Verification items for the finished model (mm, model axes). A direction names the side the tool comes from. Round coordinates to 2 decimals unless told otherwise and drop trailing zeros. Loops run counter-clockwise (first coordinate to the right, second up) from the corner with the lowest first, then second, coordinate; pieces in that order, holes last. Notation, with made-up numbers: (20, 54) -> (62, 54) arc R31 cw to (62, 79) -> close; hole circle Ø11 at (-35, -30). An arc over 180 degrees is marked (long way). Write item = value, one per line.
```python
from build123d import *

# Parameters (mm, degrees)
F4_DEPTH = 8
F2_R     = 3.171744
F5_DEPTH = 25
F0_R     = 3.171744
F6_DEPTH = 25


with BuildPart() as f4:
    # F3 (on Front) → F4 (new body)
    with BuildSketch(Plane.XZ):
        with BuildLine():
            Line((-59.009388, 95.835626), (0, -18.867213))
            Line((0, -18.867213), (59.009388, 95.835626))
            ThreePointArc((59.009388, 95.835626), (55.394876, 108.451405), (42.578131, 105.631188))
            Line((42.578131, 105.631188), (0, 23.474881))
            Line((0, 23.474881), (-42.578131, 105.631188))
            ThreePointArc((-42.578131, 105.631188), (-55.394876, 108.451405), (-59.009388, 95.835626))
        make_face()
    extrude(amount=F4_DEPTH)

    # F2 (on Front) → F5 (cut)
    with BuildSketch(Plane.XZ):
        with Locations((-50.368942, 99.972241)):
            Circle(F2_R)
        with Locations((50.368942, 99.972241)):
            Circle(F2_R)
    extrude(amount=F5_DEPTH, mode=Mode.SUBTRACT)

    # F0 (on Front) → F6 (cut)
    with BuildSketch(Plane.XZ):
        Circle(F0_R)
    extrude(amount=F6_DEPTH, mode=Mode.SUBTRACT)


solid = f4.part
```
(1) Sectioned sample at A-A, the plane z = 92. Record the cut outline in (x, y), and give its area (3 significant figures).
Filled sheet:
outline = (-57.04, -8) -> (-35.51, -8) -> (-35.51, 0) -> (-57.04, 0) -> close; (35.51, -8) -> (57.04, -8) -> (57.04, 0) -> (35.51, 0) -> close
area = 344 mm2
(2) Sectioned sample at D-D, the plane x = 6. Record the cut outline in (y, z), and give its area (3 significant figures).
Filled sheet:
outline = (-8, -7.2) -> (0, -7.2) -> (0, 35.05) -> (-8, 35.05) -> close
area = 338 mm2
(3) Sectioned sample at B-B, the plane y = -1.25. Record the cut outline in (x, z).
Filled sheet:
outline = (-59.01, 95.84) -> (0, -18.87) -> (59.01, 95.84) arc R9.58 ccw to (42.58, 105.63) -> (0, 23.47) -> (-42.58, 105.63) arc R9.58 ccw to start; hole circle Ø6.34 at (-50.37, 99.97); hole circle Ø6.34 at (0, 0); hole circle Ø6.34 at (50.37, 99.97)
(4) Go/stop test with flat-tipped pins: pin 1 Ø7.5 at (x, z) = (50.37, 99.97) entering from +Y; pin 2 Ø1.5 at (y, z) = (-6, 24) entering from +X; pin 3 Ø5 at (x, z) = (-50.37, 99.97) entering from -Y; pin 4 Ø3 at (y, z) = (-3.5, 37) entering from +X. Record where each tip stops, or that it passes through.
Filled sheet:
pin_1 = 0
pin_2 = 22.44
pin_3 = through
pin_4 = 29.51
(5) Material ranges on probe 1 along X at (y, z) = (-0.5, 35); probe 2 along X at (y, z) = (-0.75, 44); probe 3 along Z at (x, y) = (-5, -3), recorded low to high. Write a range as from..to.
Filled sheet:
probe_1 = -27.71..-5.97, 5.97..27.71
probe_2 = -32.34..-10.64, 10.64..32.34
probe_3 = -9.15..33.12
(6) Sectioned sample at C-C, the plane z = 75. Record the cut outline in (x, y).
Filled sheet:
outline = (-48.29, -8) -> (-26.7, -8) -> (-26.7, 0) -> (-48.29, 0) -> close; (26.7, -8) -> (48.29, -8) -> (48.29, 0) -> (26.7, 0) -> close
(7) Draft check along X on faces 3 (the face through (-29.92, -3.94, 39.29)), 4 (the face through (53.4, -3.9, 100.9)), 5 (the face through (-18, 0, 51)). Enter one of: released by +X, released by -X, zero draft, split by the parting line, or undercut.
Filled sheet:
face_3 = released by -X
face_4 = undercut
face_5 = zero draft
(8) Set-up check for faces 1 (the face through (21.59, -3.94, 65.13)), 2 (the face through (-2.517, -3.944, -1.93)): record each of +Z, -Z, +X, -X, +Y, -Y from which the full face is reachable in a straight line by a thin tool's end or side.
Filled sheet:
face_1 = +Z, +Y, -Y
face_2 = +Y, -Y
